from build123d import *

# Parameters (mm, degrees)
SKETCH1_W           = 565.88
SKETCH1_H           = 495.88
BOSS_EXTRUDE1_DEPTH = 3.5
SKETCH2_R           = 22.5
BOSS_EXTRUDE2_DEPTH = 15


with BuildPart() as part:
    # Sketch1 → Boss-Extrude1 (new, symmetric)
    with BuildSketch(Plane(origin=(0, 0, 0), x_dir=(1, 0, 0), z_dir=(0, 1, 0))):
        Rectangle(SKETCH1_W, SKETCH1_H)
    extrude(amount=BOSS_EXTRUDE1_DEPTH, both=True)

    # Sketch2 → Boss-Extrude2 (add)
    with BuildSketch(Plane(origin=(0, 3.5, 0), x_dir=(1, 0, 0), z_dir=(0, 1, 0))):
        with Locations(Location((70, 0, 0), (0, 0, 270))):
            Circle(SKETCH2_R)
    extrude(amount=BOSS_EXTRUDE2_DEPTH)


solid = part.part
For this review, take the finished solid that the model builds, in its own axes (mm). A direction names the side the tool comes from. Coordinates: 2 decimals unless noted, no trailing zeros. Loops run counter-clockwise (first coordinate to the right, second up) from the corner with the lowest first, then second, coordinate; pieces in that order, holes last. Notation, with made-up numbers: (-39.5, 4.5) - (-18.5, 4.5) arc R25 cw to (-18.5, 39.5) - close; hole circle Ø10 at (-38, -38). An arc over 180 degrees is marked (long way). Use a Markdown table: item, result. Add a question column.
Item 1: We need section B-B (x = 70). Give the boundary of the cut face in (y, z).
Item 2: We need section A-A (z = 0). Give the boundary of the cut face in (x, y), and give its area (3 significant figures).
Item 3: Insertion check: pin 1 Ø1 at (x, y) = (-3, 5) entering from -Z; pin 2 Ø10 at (x, z) = (122, -197) entering from +Y; pin 3 Ø8 at (y, z) = (5.5, -112) entering from -X. Each pin has a flat end and moves straight along its axis. Give the tip position at first contact, or say it passes through.
Item 4: We need section D-D (z = 86). Give the boundary of the cut face in (x, y).
Item 5: For line 1 (Y direction, x = 217.5, z = 134.5); line 2 (X direction, y = 11.5, z = -1.5); line 3 (Z direction, x = 82, y = 17.25), list the stretches that pass through material, from the lowest coordinate up.
Item 6: Tool access review of faces 1 (the face through (-4, -3.5, -3)), 2 (the face through (88.97, 10.9, 12.1)): name each direction out of +Z, -Z, +X, -X, +Y, -Y from which nothing blocks a thin tool from reaching the whole face with its end or side.
Item 7: We need section C-C (y = 11). Give the boundary of the cut face in (x, z), and give its area (3 significant figures).
Results list:
| question | item | result |
|---|---|---|
| 1 | outline | (-3.5, -247.94) - (3.5, -247.94) - (3.5, -22.5) - (18.5, -22.5) - (18.5, 22.5) - (3.5, 22.5) - (3.5, 247.94) - (-3.5, 247.94) - close |
| 2 | outline | (-282.94, -3.5) - (282.94, -3.5) - (282.94, 3.5) - (92.5, 3.5) - (92.5, 18.5) - (47.5, 18.5) - (47.5, 3.5) - (-282.94, 3.5) - close |
| 2 | area | 4,640 mm^2 |
| 3 | pin 1 | passes through |
| 3 | pin 2 | stops at y = 3.5 |
| 3 | pin 3 | stops at x = -282.94 |
| 4 | outline | (-282.94, -3.5) - (282.94, -3.5) - (282.94, 3.5) - (-282.94, 3.5) - close |
| 5 | line 1 | y = -3.5 to 3.5 |
| 5 | line 2 | x = 47.55 to 92.45 |
| 5 | line 3 | z = -19.03 to 19.03 |
| 6 | face 1 | +Z, -Z, +X, -X, -Y |
| 6 | face 2 | +Y |
| 7 | outline | circle Ø45 at (70, 0) |
| 7 | area | 1,590 mm^2 |
